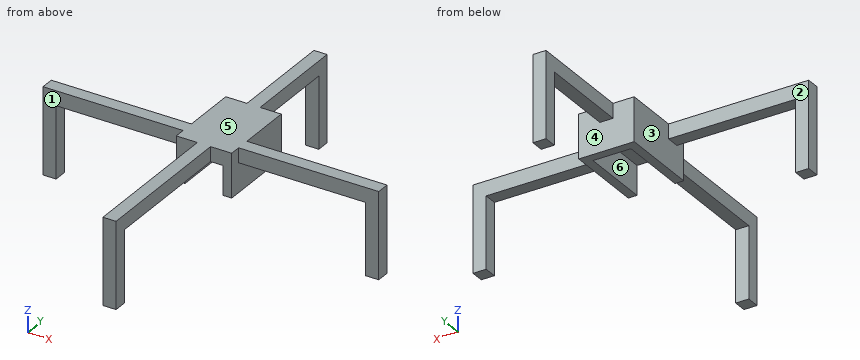
from build123d import *

# Parameters (mm, degrees)
BOSS_EXTRUDE7_DEPTH       = 2.25
BOSS_EXTRUDE7_DEPTH_BACK  = 2.25
BOSS_EXTRUDE10_DEPTH      = 10
BOSS_EXTRUDE12_DEPTH      = 2.25
BOSS_EXTRUDE12_DEPTH_BACK = 2.25
SKETCH11_W                = 19
SKETCH11_H                = 27
BOSS_EXTRUDE13_DEPTH      = 5
SKETCH12_W                = 148.824805779
SKETCH12_H                = 155.89300236
CUT_EXTRUDE1_DEPTH        = 2


with BuildPart() as part:
    # Sketch8 → Boss-Extrude7 (new body, two sides)
    with BuildSketch(Plane(origin=(0, 2.5, 0), x_dir=(1, 0, 0), z_dir=(0, 1, 0))) as boss_extrude7_sk:
        Polygon((-57.5, -4), (57.5, -4), (57.5, 27.5), (53, 27.5), (53, 1), (-53, 1), (-53, 27.5), (-57.5, 27.5), align=None)
    extrude(amount=BOSS_EXTRUDE7_DEPTH)
    extrude(boss_extrude7_sk.sketch, amount=-BOSS_EXTRUDE7_DEPTH_BACK)

    # Sketch10 → Boss-Extrude10 (add)
    with BuildSketch(Plane(origin=(0, 0, -1), x_dir=(-1, 0, 0), z_dir=(0, 0, -1))):
        Polygon((6.5, 20.5), (-6.5, 20.5), (-6.5, -2.5), (-6.5, -3.5), (-9.5, -3.5), (-9.5, -2.5), (-9.5, 23.5), (9.5, 23.5), (9.5, -2.5), (9.5, -3.5), (6.5, -3.5), (6.5, -2.5), align=None)
    extrude(amount=BOSS_EXTRUDE10_DEPTH)

    # Sketch6 → Boss-Extrude12 (add, two sides)
    with BuildSketch(Plane(origin=(0, 0, 0), x_dir=(0, 0, -1), z_dir=(1, 0, 0))) as boss_extrude12_sk:
        Polygon((27.5, 55.5), (1, 55.5), (1, -50.5), (27.5, -50.5), (27.5, -55), (-4, -55), (-4, 60), (27.5, 60), align=None)
    extrude(amount=BOSS_EXTRUDE12_DEPTH)
    extrude(boss_extrude12_sk.sketch, amount=-BOSS_EXTRUDE12_DEPTH_BACK)

    # Sketch11 → Boss-Extrude13 (add)
    with BuildSketch(Plane.XY.offset(-1)):
        with Locations((0, 10)):
            Rectangle(SKETCH11_W, SKETCH11_H)
    extrude(amount=BOSS_EXTRUDE13_DEPTH)

    # Sketch12 → Cut-Extrude1 (cut)
    with BuildSketch(Plane(origin=(0, 0, -27.5), x_dir=(-1, 0, 0), z_dir=(0, 0, -1))):
        with Locations((-7.264535374, 8.488333214)):
            Rectangle(SKETCH12_W, SKETCH12_H)
    extrude(amount=-CUT_EXTRUDE1_DEPTH, mode=Mode.SUBTRACT)


solid = part.part
Work out the finished part from the listing and answer in its coordinate system (mm). Face numbers are marked on the shaded views. A direction names the side the tool comes from. Give positions to 0.01 mm unless a question says otherwise; leave off trailing zeros. Write each loop counter-clockwise with the first axis right and the second up, starting at its lowest first coordinate (ties: lowest second). Pieces come first, ordered by that corner, then holes.
Q1. Given pin 1 (5.5 mm diameter, centred on x = -2, y = 4, fed in from -Z); pin 2 (15 mm diameter, centred on y = 35.5, z = -11, fed in from -X); pin 3 (4.5 mm diameter, centred on y = 16, z = -5, fed in from +X); pin 4 (3.5 mm diameter, centred on x = -7, z = -6.5, fed in from -Y), each flat-ended and moving along its own axis, determine where each tip first touches the part or whether it passes through.
Answer:
pin 1: stops at z = -1
pin 2: passes through
pin 3: stops at x = 9.5
pin 4: stops at y = -3.5
Q2. The part is cut by section B-B on z = -23. Give the vertices of the cut face in (x, y), and give its area (3 significant figures).
Answer:
outline: (-57.5, 0.25) - (-53, 0.25) - (-53, 4.75) - (-57.5, 4.75) - close; (-2.25, -55) - (2.25, -55) - (2.25, -50.5) - (-2.25, -50.5) - close; (-2.25, 55.5) - (2.25, 55.5) - (2.25, 60) - (-2.25, 60) - close; (53, 0.25) - (57.5, 0.25) - (57.5, 4.75) - (53, 4.75) - close
area: 81.0 mm2
Q3. The part is cut by section D-D on y = -8.5. Give the vertices of the cut face in (x, z).
Answer:
outline: (-2.25, -1) - (2.25, -1) - (2.25, 4) - (-2.25, 4) - close
Q4. The part is cut by section C-C on x = -18. Give the vertices of the cut face in (y, z).
Answer:
outline: (0.25, -1) - (4.75, -1) - (4.75, 4) - (0.25, 4) - close
Q5. For a pull along Y with two mould halves and no side action, classify the marked faces 1, 2, 3 and 4 as released by +Y, released by -Y, zero draft, split by the parting line, or undercut.
Answer:
face 1: released by -Y
face 2: released by +Y
face 3: zero draft
face 4: undercut
Q6. The part is cut by section A-A on z = -4. Give the vertices of the cut face in (x, y), and give its area (3 significant figures).
Answer:
outline: (-57.5, 0.25) - (-53, 0.25) - (-53, 4.75) - (-57.5, 4.75) - close; (-9.5, -3.5) - (-6.5, -3.5) - (-6.5, 20.5) - (6.5, 20.5) - (6.5, -3.5) - (9.5, -3.5) - (9.5, 23.5) - (-9.5, 23.5) - close; (-2.25, -55) - (2.25, -55) - (2.25, -50.5) - (-2.25, -50.5) - close; (-2.25, 55.5) - (2.25, 55.5) - (2.25, 60) - (-2.25, 60) - close; (53, 0.25) - (57.5, 0.25) - (57.5, 4.75) - (53, 4.75) - close
area: 282 mm2
Q7. A tool of negligible diameter and unlimited length cuts with its end or side. For the marked faces 5 and 6, from which of +Z, -Z, +X, -X, +Y, -Y can it reach the whole face along a straight path? Write none if from no direction.
Answer:
face 5: +Z, +X, -X, +Y, -Y
face 6: -Z, -Y
Q8. Straight lines are drawn through the part: L1, parallel to X at y = 9.5, z = -2.5; L2, parallel to Z at x = -1.5, y = 6.5; L3, parallel to Y at x = 17, z = -0.75. For each, find the intervals that lie inside material, in ascending order.
Answer:
L1: x = -9.5 to -6.5, 6.5 to 9.5
L2: z = -1 to 4
L3: y = 0.25 to 4.75
